Autodesk Inventor part; units mm, degrees
ref_plane "IDS_WORKPLANE{1}" through (-3.81, 0, 0) normal (1, 0, 0) x (0, 0, -1)
ref_plane "Work Plane2" through (1.4224, 0, 0) normal (0, 0, -1) x (1, 0, 0)
ref_plane "YZ Plane" through (0, 0, 0) normal (1, 0, 0) x (0, 1, 0)
sketch "Sketch1" plane through (0, 0, 0) normal (0, 0, 1) x (1, 0, 0)
  line L0 (-3.81, 0) -> (44.45, 0)
  line L1 (44.45, 0) -> (44.45, 3.175)
  line L2 (44.45, 3.175) -> (0, 3.175)
  line L3 (0, 3.175) -> (0, 7.2771)
  line L4 (-14.4263, 0) -> (54.2627, 0)
  line L5 (0, -1.5301) -> (0, 9.1803)
  line L6 (0, 7.2771) -> (-0.4307, 7.2771)
  arc A0 (-0.4307, 7.2771) -> (-3.81, 0) centre (5.715, 0) ccw
  dimension "d0" = 44.45
  dimension "d3" = 3.81
  dimension "d4" = 6.35
  dimension "d9" = 14.5542
  dimension "d10" = 0
  dimension "d13" = 9.525
revolve "Body" add sketch "Sketch1" angle 360 about axis through (-3.81, 0, 0) along (1, 0, 0)
ref_plane "IDS_WORKPLANE{1}" through (-3.81, 0, 0) normal (1, 0, 0) x (0, 0, -1)
sketch "Sketch2" plane through (-3.81, 0, 0) normal (1, 0, 0) x (0, 0, -1)
  circle A0 centre (0, 0) radius 7.2771
  line L0 (0, -10.1879) -> (0, 10.1879)
  line L1 (10.1879, 0) -> (-10.1879, 0)
  line L2 (-7.2771, 0.9525) -> (7.2771, 0.9525)
  line L3 (7.2771, 0.9525) -> (7.2771, -0.9525)
  line L4 (7.2771, -0.9525) -> (-7.2771, -0.9525)
  line L5 (-7.2771, -0.9525) -> (-7.2771, 0.9525)
  line L6 (-7.2771, 0) -> (7.2771, 0) construction
  line L7 (0, 0.9525) -> (0, -0.9525) construction
  dimension "d15" = 1.905
extrude "Slot" cut sketch "Sketch2" along normal blind 2.2098 contours L1 L0 L2 A0 | L3 L4 A0 | A0 L4 L0 L1 | A0 L2 L3 | L1 A0 L2 L0 | L0 L4 A0 L1 | L5 L2 A0 | A0 L4 L5
thread "Thread"
sketch "Sketch3" plane through (0, 0, 0) normal (0, 0, 1) x (1, 0, 0)
  line L0 (44.45, 0) -> (44.45, 3.175)
  line L1 (-3.81, 0) -> (44.45, 0)
  arc A0 (44.45, 0) -> (41.275, 3.175) centre (41.275, 0) ccw
  line L2 (44.45, -3.175) -> (44.45, 3.175)
  line L3 (41.275, 3.175) -> (41.275, 0)
  line L4 (41.275, 0) -> (44.45, 0)
  line L5 (0, 3.175) -> (44.45, 3.175)
revolve "Fillet" cut sketch "Sketch3" angle 360 about axis through (-3.81, 0, 0) along (1, 0, 0) contours A0 L5 L0
ref_plane "Work Plane2" through (1.4224, 0, 0) normal (0, 0, -1) x (1, 0, 0)
equation "\"d0\" = NLG"
equation "\"d3\" = KOH"
equation "\"d4\" = GD"
equation "\"d9\" = KOD"
equation "\"d13\" = KR"
equation "\"d15\" = SBR"
equation "\"d16\" = STI"
equation "\"d11\" = GEL"
equation "\"GD\" = NND"
equation "\"NLG\" = 44.45"
equation "\"GEL\" = 37.7825"
equation "\"KOD\" = 14.5542"
equation "\"KOH\" = 3.81"
equation "\"SBR\" = 1.905"
equation "\"STI\" = 2.2098"
equation "\"KEWI\" = 0"
equation "\"KR\" = 9.525"
equation "\"d14\" = -KOH"
equation "\"GUL\" = GAL"
equation "\"SPD\" = 5.44322"
equation "\"THREADDIA\" = 6.35"
equation "\"TOA\" = 30deg"
equation "\"BDM\" = NND"
equation "\"NND\" = 6.35"
equation "\"GAL\" = 0.45339"
equation "\"GD1\" = 5.44322"
properties part number "ANSI B18.6.3 - 1/4 - 28 - 1 3/4, STHMSI" material "Steel, Mild"
Could you check a few things on this model? Use its own coordinates, in mm. A direction names the side the tool comes from. Round coordinates to 2 decimals unless told otherwise and drop trailing zeros. Loops run counter-clockwise (first coordinate to the right, second up) from the corner with the lowest first, then second, coordinate; pieces in that order, holes last. Notation, with made-up numbers: (23.5, 76.5) - (33.5, 76.5) arc R20 cw to (33.5, 97.5) - close; hole circle Ø10 at (79.5, -28). An arc over 180 degrees is marked (long way). Answer in a Markdown table with one row per item. Add a question column.
(1) I need wall thicknesses on line 1 along X through (y, z) = (-2.25, -2.75); line 2 along X through (y, z) = (-2.75, -4.75); line 3 along Z through (x, y) = (16, 2). Which ranges of each line are inside material? Lowest first, please.
(2) I'm going to push flat-ended pins straight in: pin 1 (2.5 mm diameter, centred on x = -2.5, z = 1, fed in from +Y); pin 2 (4 mm diameter, centred on y = 2.5, z = 3, fed in from +X); pin 3 (3 mm diameter, centred on y = 4, z = -2.5, fed in from +X). Where does each tip first touch, or does it pass through?
(3) For faces 4 (the face through (-2, 0.952, 0)), 5 (the face through (-0.22, 6.94, -2.19)), which set-ups out of +Z, -Z, +X, -X, +Y, -Y let a thin tool reach every point of the face, with its end or its side?
(4) If we mould it in two halves opening along Y, with no side actions, what happens to faces 1 (the face through (20.35, -0.69, 3.1)), 2 (the face through (-2, -0.952, 0)), 3 (the face through (0, 3, -2))? For each: pulls with the +Y half, pulls with the -Y half, needs draft (parallel to the pull), parting line crosses it, or undercut.
(5) If we section it at A-A (x = 38): Please give me the cut outline in (y, z) (3 decimals).
Model answer:
| question | item | result |
|---|---|---|
| 1 | line 1 | x = -3.12 to 0 |
| 1 | line 2 | x = -2.07 to 0 |
| 1 | line 3 | z = -2.47 to 2.47 |
| 2 | pin 1 | stops at y = 6.43 |
| 2 | pin 2 | stops at x = 43.81 |
| 2 | pin 3 | stops at x = 0 |
| 3 | face 4 | +Z, -Z, -X |
| 3 | face 5 | +X, -X |
| 4 | face 1 | parting line crosses it |
| 4 | face 2 | undercut |
| 4 | face 3 | needs draft |
| 5 | outline | circle Ø6.35 at (0, 0) |
